Design review of the part built by this model. Coordinates are the model's own, in mm. A direction names the side the tool comes from. Round coordinates to 2 decimals unless told otherwise and drop trailing zeros. Order: outer loops, then holes, each group sorted by start corner. A loop starts at its lowest first (then second) coordinate and runs counter-clockwise, first axis right, second up. Notation, with made-up numbers: M -33,-36.5 L 22,-36.5 A19 ccw 22,-13.5 Z; hole C 20.25,-33 d1. An arc over 180 degrees is marked long. Use a Markdown table: item, result. Add a question column.
(1) To check wall thickness, follow probe 1 along Y at (x, z) = (-6.6, 0); probe 2 along X at (y, z) = (29.3, 0); probe 3 along Z at (x, y) = (-8, 6). State the ranges of each line that lie inside material, in increasing order. Write a range as from..to.
(2) Machinability: for faces 1 (the face through (3.2, 29.5, 10)), 2 (the face through (6, 30, -9)), 3 (the face through (0, 7, -4.5)), which of the approach directions +Z, -Z, +X, -X, +Y, -Y give a long, thin tool a straight path to every point of the face, cutting with its end or side? Answer none if there is none.
(3) For pin 1 (1 mm diameter, centred on y = 10.5, z = 8, fed in from -X); pin 2 (7 mm diameter, centred on x = 0.5, y = 10.5, fed in from -Z); pin 3 (4 mm diameter, centred on y = 6, z = 0, fed in from -X); pin 4 (2.5 mm diameter, centred on y = 10.5, z = 1.5, fed in from +X), all flat-tipped, find the tip position at first contact; note any pin that passes through.
(4) The part is to be moulded in two halves that separate along Y. For faces 4 (the face through (-7.91, 27.042, -10.316)), 5 (the face through (0, 15, 0)), 6 (the face through (-5, 29, 5)), 7 (the face through (7.22, 8.48, 0.33)), say which applies: released by +Y, released by -Y, zero draft, split by the parting line, or undercut.
(5) Take a section at C-C (x = -3). Write out the cut boundary in (y, z), then the cut area to 3 significant figures.
(6) Take a section at D-D (z = 6.75). Write out the cut boundary in (x, y).
(7) Take a section at B-B (y = 6). Write out the cut boundary in (x, z), then the cut area to 3 significant figures.
(8) Take a section at A-A (z = 1). Write out the cut boundary in (x, y), then the cut area to 3 significant figures.
```python
from build123d import *

# Parameters (mm, degrees)
SKETCH_1_R               = 10
EXTRUDE_1_DEPTH          = 30
SKETCH_2_R               = 13
EXTRUDE_2_DEPTH          = 6
CUT_EXTRUDE_1_DEPTH      = 36.185224172
CUT_EXTRUDE_1_DEPTH_BACK = 36.185224172
SKETCH_3_R               = 2.5
SKETCH_4_W               = 9
SKETCH_4_H               = 9
CUT_EXTRUDE_2_DEPTH      = 15
SKETCH_6_R               = 10.5
CUT_EXTRUDE_3_DEPTH      = 1


with BuildPart() as part:
    # 草图1 → 凸台-拉伸1 (new body)
    with BuildSketch(Plane(origin=(0, 0, 0), x_dir=(1, 0, 0), z_dir=(0, 1, 0))):
        with Locations(Location((0, 0, 0), (0, 0, 270))):
            Circle(SKETCH_1_R)
    extrude(amount=EXTRUDE_1_DEPTH)

    # 草图2 → 凸台-拉伸2 (add)
    with BuildSketch(Plane(origin=(0, 30, 0), x_dir=(1, 0, 0), z_dir=(0, 1, 0))):
        with Locations(Location((0, 0, 0), (0, 0, 270))):
            Circle(SKETCH_2_R)
    extrude(amount=-EXTRUDE_2_DEPTH)

    # 草图3 → 切除-拉伸1 (cut, two sides: drawn at the far end of the back side and taken through both)
    with BuildSketch(Plane(origin=(0, 0, 0), x_dir=(0, 0, -1), z_dir=(1, 0, 0)).offset(-CUT_EXTRUDE_1_DEPTH_BACK)):
        with Locations((0, 6)):
            Circle(SKETCH_3_R)
    extrude(amount=CUT_EXTRUDE_1_DEPTH + CUT_EXTRUDE_1_DEPTH_BACK, mode=Mode.SUBTRACT)

    # 草图4 → 切除-拉伸2 (cut)
    with BuildSketch(Plane(origin=(0, 0, 0), x_dir=(-1, 0, 0), z_dir=(0, -1, 0))):
        Rectangle(SKETCH_4_W, SKETCH_4_H)
    extrude(amount=-CUT_EXTRUDE_2_DEPTH, mode=Mode.SUBTRACT)

    # 草图5 → 切除-旋转1 (revolve, cut)
    with BuildSketch(Plane.XY):
        with BuildLine():
            Line((0, 33.394315723), (0, 21.394315723))
            ThreePointArc((0, 21.394315723), (6, 27.394315723), (0, 33.394315723))
        make_face()
    revolve(axis=Axis((0, 37.883813042, 0), (0, -1, 0)), mode=Mode.SUBTRACT)

    # 草图6 → 切除-拉伸3 (cut)
    with BuildSketch(Plane(origin=(0, 30, 0), x_dir=(1, 0, 0), z_dir=(0, 1, 0))):
        with Locations(Location((0, 0, 0), (0, 0, 270))):
            Circle(SKETCH_6_R)
    extrude(amount=-CUT_EXTRUDE_3_DEPTH, mode=Mode.SUBTRACT)


solid = part.part
```
Verdict:
| question | item | result |
|---|---|---|
| 1 | probe 1 | y = 0..3.5, 8.5..29 |
| 1 | probe 2 | x = -13..-10.5, 10.5..13 |
| 1 | probe 3 | z = -6..-2.5, 2.5..6 |
| 2 | face 1 | +Y |
| 2 | face 2 | +Z, -Z, +X, -X, +Y |
| 2 | face 3 | -Y |
| 3 | pin 1 | stops at x = -6.61 |
| 3 | pin 2 | stops at z = -10 |
| 3 | pin 3 | passes through |
| 3 | pin 4 | stops at x = 10 |
| 4 | face 4 | zero draft |
| 4 | face 5 | released by -Y |
| 4 | face 6 | released by +Y |
| 4 | face 7 | undercut |
| 5 | outline | M 0,-9.54 L 24,-9.54 L 24,-12.65 L 30,-12.65 L 30,-10.06 L 29,-10.06 L 29,-4.94 A5.2 cw long 29,4.94 L 29,10.06 L 30,10.06 L 30,12.65 L 24,12.65 L 24,9.54 L 0,9.54 L 0,4.5 L 15,4.5 L 15,-4.5 L 0,-4.5 Z |
| 5 | area | 396 mm^2 |
| 6 | outline | M -11.11,24 L -7.38,24 L -7.38,0 L 7.38,0 L 7.38,24 L 11.11,24 L 11.11,30 L 8.04,30 L 8.04,29 L -8.04,29 L -8.04,30 L -11.11,30 Z |
| 7 | outline | M -9.68,-2.5 A10 ccw 9.68,-2.5 L 4.5,-2.5 L 4.5,-4.5 L -4.5,-4.5 L -4.5,-2.5 Z; M -9.68,2.5 L -4.5,2.5 L -4.5,4.5 L 4.5,4.5 L 4.5,2.5 L 9.68,2.5 A10 ccw Z |
| 7 | area | 179 mm^2 |
| 8 | outline | M -12.96,24 L -9.95,24 L -9.95,8.29 L -4.5,8.29 L -4.5,15 L 4.5,15 L 4.5,8.29 L 9.95,8.29 L 9.95,24 L 12.96,24 L 12.96,30 L 10.45,30 L 10.45,29 L 5.69,29 A5.92 cw long -5.69,29 L -10.45,29 L -10.45,30 L -12.96,30 Z; M -9.95,0 L -4.5,0 L -4.5,3.71 L -9.95,3.71 Z; M 4.5,0 L 9.95,0 L 9.95,3.71 L 4.5,3.71 Z |
| 8 | area | 354 mm^2 |
